Design review of the part built by this model. Coordinates are the model's own, in mm. Give positions to 0.01 mm unless a question says otherwise; leave off trailing zeros. Loops run counter-clockwise (first coordinate to the right, second up) from the corner with the lowest first, then second, coordinate; pieces in that order, holes last. Notation, with made-up numbers: (-32, -13.75) -> (-4, -13.75) arc R31 cw to (-4, 22.25) -> close; hole circle Ø9 at (88, -32). An arc over 180 degrees is marked (long way). Answer in a Markdown table with one row per item. Add a question column.
(1) For line 1 (Z direction, x = 1.2, y = -120.2); line 2 (Y direction, x = 1.7, z = -216.75); line 3 (Z direction, x = 1.35, y = 74), list the stretches that pass through material, from the lowest coordinate up.
(2) Consider section C-C on x = 1.5. Count the separate pieces of the cut face and the enclosed holes in it, then the cut area to 3 significant figures.
(3) For pin 1 (8 mm diameter, centred on y = -25, z = -216.75, fed in from -X); pin 2 (1 mm diameter, centred on x = 0.5, y = -47, fed in from +Z); pin 3 (1 mm diameter, centred on x = 1.5, y = 101, fed in from +Z); pin 4 (1 mm diameter, centred on x = 1.5, z = -155.5, fed in from +Y), all flat-tipped, find the tip position at first contact; note any pin that passes through.
(4) Draft analysis for pull direction Y (two halves, no side actions). For faces 1 (the flat face through (1.565, 23.665, -389.587)), 2 (the flat face through (1.57, -16.66, -150.86)), 3 (the flat face through (1.565, 0.768, -139.304)), 4 (the flat face through (0, -35, -255)), state which applies: +Y half, -Y half, draft (parallel to the pull), parting line (faces both ways), or undercut.
(5) Consider section D-D on y = 98. Write out the cut boundary in (x, z) (3 decimals).
(6) Consider section B-B on z = -279. Write out the cut boundary in (x, y) (3 decimals), then the cut area to 3 significant figures.
Autodesk Inventor part; units mm, degrees
ref_plane "YZ Plane" through (0, 0, 0) normal (1, 0, 0) x (0, 1, 0)
ref_plane "XZ Plane" through (0, 0, 0) normal (0, 1, 0) x (-1, 0, 0)
ref_plane "XY Plane" through (0, 0, 0) normal (0, 0, 1) x (1, 0, 0)
sketch "Sketch1" plane through (0, 0, 0) normal (1, 0, 0) x (0, 1, 0)
  line L0 (-120.8333, -99.25) -> (-47.8333, -99.25)
  line L1 (-120.2, -86.75) -> (-120.2, -99.25) construction
  line L2 (0, -198.5) -> (40, -198.5) construction
  line L3 (40, -198.5) -> (40, -265) construction
  line L4 (40, -265) -> (0, -265) construction
  line L5 (0, -265) -> (0, -198.5) construction
  line L6 (0, -265) -> (40, -265) construction
  line L7 (40, -265) -> (40, -285) construction
  line L8 (40, -285) -> (0, -285)
  line L9 (0, -285) -> (0, -265) construction
  line L10 (0, -198.5) -> (40, -198.5) construction
  line L11 (40, -198.5) -> (40, -178.5) construction
  line L12 (40, -178.5) -> (0, -178.5) construction
  line L13 (0, -178.5) -> (0, -198.5) construction
  line L14 (48.2, -259.95) -> (-8.2, -259.95) construction
  line L15 (-8.2, -259.95) -> (-8.2, -203.55) construction
  line L16 (-8.2, -203.55) -> (48.2, -203.55) construction
  line L17 (48.2, -203.55) -> (48.2, -259.95) construction
  line L18 (48.2, -231.75) -> (-8.2, -231.75) construction
  line L19 (40, -231.75) -> (0, -231.75) construction
  line L20 (43.57, -255.32) -> (-3.57, -255.32) construction
  line L21 (-3.57, -255.32) -> (-3.57, -208.18) construction
  line L22 (-3.57, -208.18) -> (43.57, -208.18) construction
  line L23 (43.57, -208.18) -> (43.57, -255.32) construction
  line L24 (43.57, -255.32) -> (48.2, -255.32) construction
  line L25 (43.57, -255.32) -> (43.57, -259.95) construction
  line L26 (-3.57, -208.18) -> (-8.2, -208.18) construction
  line L27 (-3.57, -208.18) -> (-3.57, -203.55) construction
  line L28 (40, -188.5) -> (0, -188.5) construction
  line L29 (40, -275) -> (0, -275) construction
  circle A0 centre (30, -275) radius 2.1
  circle A1 centre (10, -275) radius 2.1
  circle A2 centre (30, -188.5) radius 2.1
  circle A3 centre (10, -188.5) radius 2.1
  circle A4 centre (43.57, -255.32) radius 2.6
  circle A5 centre (43.57, -208.18) radius 2.6
  circle A6 centre (-3.57, -208.18) radius 2.6
  circle A7 centre (-3.57, -255.32) radius 2.6
  circle A8 centre (20, -231.75) radius 19.15
  circle A9 centre (-25, -216.75) radius 11.08 construction
  circle A10 centre (-25, -216.75) radius 13 construction
  circle A11 centre (-25, -216.75) radius 2.5
  line L30 (-60, -351.75) -> (-60, -111.75) construction
  circle A12 centre (-60, -111.75) radius 2.6
  circle A13 centre (-60, -351.75) radius 2.6
  line L31 (-120.2, -351.75) -> (-120.2, -111.75) construction
  circle A14 centre (-120.2, -111.75) radius 2.6
  circle A15 centre (-120.2, -351.75) radius 2.6
  circle A16 centre (-60, -111.75) radius 12 construction
  circle A17 centre (-120.2, -111.75) radius 12 construction
  circle A18 centre (-120.2, -351.75) radius 12 construction
  circle A19 centre (-60, -351.75) radius 12 construction
  circle A20 centre (-25, -246.75) radius 2.5
  circle A21 centre (-25, -246.75) radius 11.08 construction
  circle A22 centre (-25, -246.75) radius 13 construction
  circle A23 centre (20, -231.75) radius 11.08 construction
  circle A24 centre (20, -231.75) radius 13 construction
  line L32 (-23.1873, -227.6807) -> (18.1873, -220.8193) construction
  line L33 (18.1873, -242.6807) -> (-23.1873, -235.8193) construction
  line L34 (-47.8333, -364.25) -> (-120.8333, -364.25)
  line L35 (-132.8333, -352.25) -> (-132.8333, -111.25)
  line L36 (-60, -351.75) -> (-120.2, -351.75) construction
  line L37 (-120.2, -111.75) -> (-60, -111.75) construction
  line L38 (-60, -351.75) -> (-60, -364.25) construction
  line L39 (-120.2, -111.75) -> (-120.2, -99.25) construction
  line L40 (48.3276, -178.5) -> (48.3276, -285)
  line L41 (17.6122, -285) -> (40, -285) construction
  arc A25 (-132.8333, -352.25) -> (-120.8333, -364.25) centre (-120.8333, -352.25) ccw
  arc A26 (-120.8333, -99.25) -> (-132.8333, -111.25) centre (-120.8333, -111.25) ccw
  line L42 (48.3276, -178.5) -> (-47.8333, -99.25)
  line L43 (-47.8333, -364.25) -> (-47.8333, -99.25) construction
  line L44 (-120.2, -111.75) -> (-132.8333, -111.75) construction
  line L45 (-60, -351.75) -> (-47.8333, -351.75) construction
  line L46 (-36.08, -246.75) -> (-36.08, -485.113) construction
  line L47 (-47.8333, -344.25) -> (-47.8333, -285)
  line L48 (-47.8333, -285) -> (16.8804, -285)
  line L49 (-47.8333, -125.1668) -> (16.8804, -178.5)
  line L50 (-47.8333, -178.5) -> (16.8804, -178.5)
  line L51 (-47.8333, -125.1668) -> (-47.8333, -178.5)
  line L52 (48.3276, -285) -> (48.3276, -364.25)
  line L53 (48.3276, -364.25) -> (-47.8333, -364.25)
  line L54 (-47.8333, -344.25) -> (28.3276, -344.25)
  line L55 (28.3276, -344.25) -> (28.3276, -285)
  line L56 (-47.8333, -344.25) -> (28.3276, -285) construction
  line L57 (-39.6904, -344.25) -> (28.3276, -291.3349)
  line L58 (-47.8333, -337.9151) -> (20.1847, -285)
  line L59 (48.3276, -414.25) -> (124.3276, -414.25)
  line L60 (124.3276, -414.25) -> (124.3276, -364.25)
  line L61 (124.3276, -364.25) -> (48.3276, -364.25)
  line L62 (48.3276, -364.25) -> (48.3276, -414.25)
  line L63 (48.3276, -414.25) -> (-1.6724, -364.25)
  line L64 (98.3276, -364.25) -> (48.3276, -314.25)
  point P0 (-132.8333, -99.25)
  point P1 (28.3276, 86.5)
  point P2 (0, 86.5)
  point P3 (20.1847, 86.5)
  point P4 (20.1847, 86.5)
  point P5 (0, 86.5)
  point P6 (-132.8333, -364.25)
  point P7 (-47.8333, -338.3332)
  point P8 (0, -285)
  point P9 (48.3276, -364.25)
  dimension "d222" = 85
  dimension "d242" = 76
  dimension "d243" = 50
  dimension "d244" = 45
  dimension "d245" = 50
  dimension "d246" = 45
extrude "Extrusion1" add sketch "Sketch1" along normal blind 3.175 contours L0 L42 L40 L52 L53 L34 A25 L35 A26 | L62 L63 L53 | L61 L60 L59 L62 | L55 L57 L54 L47 L58 L8 | L58 L47 L48 L8 | L55 L54 L57 | A0 | A1 | A2 | A3 | A4 | A5 | A6 | A7 | A8
sketch "Sketch6" plane through (3.175, 0, 0) normal (1, 0, 0) x (0, 0, -1)
  line L0 (125.1668, -47.8333) -> (178.5, 16.8804)
  line L1 (291.3349, 28.3276) -> (344.25, 28.3276)
  line L2 (159.4204, -6.2705) -> (143.9864, 6.4492) construction
  line L3 (178.5, 48.3276) -> (99.25, -47.8333) construction
  line L4 (291.3349, 28.3276) -> (344.25, 28.3276) construction
  line L5 (317.7924, 28.3276) -> (317.7924, 48.3276) construction
  line L6 (364.25, 48.3276) -> (178.5, 48.3276) construction
  line L7 (151.7034, 0.0893) -> (161.2432, 11.6648) construction
  line L8 (151.7034, 0.0893) -> (142.1636, -11.4861) construction
  line L9 (317.7924, 38.3276) -> (302.7924, 38.3276) construction
  line L10 (317.7924, 38.3276) -> (332.7924, 38.3276) construction
  circle A0 centre (332.7924, 38.3276) radius 2.6
  circle A1 centre (302.7924, 38.3276) radius 2.6
  circle A2 centre (161.2432, 11.6648) radius 2.6
  circle A3 centre (142.1636, -11.4861) radius 2.6
  point P0 (414.25, 48.3276)
  point P1 (314.25, 48.3276)
  dimension "d233" = 15
  dimension "d234" = 15
  dimension "d235" = 15
  dimension "d236" = 15
  dimension "d237" = 5.2
  dimension "d238" = 5.2
  dimension "d239" = 5.2
  dimension "d240" = 5.2
  dimension "d241" = 30
extrude "Extrusion6" cut sketch "Sketch6" against normal through all
fillet "Fillet2" radius 3.175 5 edges at (1.5875, -47.8333, -125.1668) (1.5875, -47.8333, -178.5) (1.5875, 16.8804, -178.5) (1.5875, -47.8333, -99.25) (1.5875, 48.3276, -178.5)
fillet "Fillet3" radius 3.175 5 edges at (1.5875, 48.3276, -364.25) (1.5875, -1.6724, -364.25) (1.5875, 48.3276, -414.25) (1.5875, 124.3276, -414.25) (1.5875, 124.3276, -364.25)
sketch "Sketch7" plane through (3.175, 0, 0) normal (1, 0, 0) x (0, 0, -1)
  line L0 (414.25, 49.6427) -> (414.25, 121.1526) construction
  line L1 (414.25, 121.5776) -> (394.25, 121.5776) construction
  line L2 (394.25, 121.5776) -> (394.25, 71.5776) construction
  line L3 (394.25, 71.5776) -> (414.25, 71.5776) construction
  line L4 (414.25, 71.5776) -> (414.25, 121.5776) construction
  line L5 (404.25, 121.5776) -> (404.25, 71.5776) construction
  circle A0 centre (404.25, 106.5776) radius 2.6
  circle A1 centre (404.25, 86.5776) radius 2.6
  line L6 (411.075, 124.3276) -> (367.425, 124.3276)
  point P0 (0, 0)
  dimension "d248" = 20
  dimension "d249" = 50
  dimension "d250" = 5.2
  dimension "d251" = 5.2
  dimension "d252" = 15
  dimension "d253" = 15
  dimension "d256" = 2.75
extrude "Extrusion7" cut sketch "Sketch7" against normal up to next
sketch "Sketch8" plane through (3.175, 0, 0) normal (1, 0, 0) x (0, 0, -1)
  line L0 (302.7924, 28.3276) -> (332.7924, 28.3276) construction
  line L1 (332.7924, 28.3276) -> (332.7924, -26.6724) construction
  line L2 (332.7924, -26.6724) -> (302.7924, -26.6724) construction
  line L3 (302.7924, -26.6724) -> (302.7924, 28.3276) construction
  circle A0 centre (332.7924, 38.3276) radius 2.6
  circle A1 centre (302.7924, 38.3276) radius 2.6
  line L4 (332.7924, 38.3276) -> (302.7924, 38.3276) construction
  line L5 (317.7924, 38.3276) -> (317.7924, 28.3276) construction
  line L6 (328.7924, -26.6724) -> (306.7924, -26.6724) construction
  line L7 (306.7924, -26.6724) -> (306.7924, -6.6724) construction
  line L8 (306.7924, -6.6724) -> (328.7924, -6.6724) construction
  line L9 (328.7924, -6.6724) -> (328.7924, -26.6724) construction
  line L10 (312.7924, -11.6724) -> (322.7924, -11.6724) construction
  line L11 (322.7924, -11.6724) -> (322.7924, -21.6724) construction
  line L12 (322.7924, -21.6724) -> (312.7924, -21.6724) construction
  line L13 (312.7924, -21.6724) -> (312.7924, -11.6724) construction
  circle A2 centre (312.7924, -11.6724) radius 2.6
  circle A3 centre (322.7924, -21.6724) radius 2.6
  point P0 (0, 0)
  dimension "d257" = 30
  dimension "d258" = 55
  dimension "d259" = 10
  dimension "d260" = 22
  dimension "d261" = 20
  dimension "d262" = 4
  dimension "d263" = 10
  dimension "d264" = 10
  dimension "d265" = 5
  dimension "d266" = 6
  dimension "d267" = 5.2
  dimension "d268" = 5.2
extrude "Extrusion8" cut sketch "Sketch8" against normal up to next contours A2 | A3
sketch "Sketch9" plane through (3.175, 0, 0) normal (1, 0, 0) x (0, 0, -1)
  line L0 (45.8374, 19.9996) -> (577.1226, 19.9996) construction
  line L1 (361.075, 48.3276) -> (179.9977, 48.3276) construction
  line L2 (231.7502, 111.484) -> (231.7502, -169.9488) construction
  circle A0 centre (161.2432, 11.6648) radius 2.6
  circle A1 centre (231.7502, 19.9996) radius 3.5
  circle A2 centre (251.7502, 19.9996) radius 2.6
  circle A3 centre (211.7502, 19.9996) radius 2.6
  point P0 (0, 0)
  dimension "d271" = 28.328
  dimension "d272" = 70.507
  dimension "d273" = 7
  dimension "d274" = 5.2
  dimension "d275" = 20
  dimension "d276" = 5.2
  dimension "d277" = 20
extrude "Extrusion9" cut sketch "Sketch9" against normal up to next contours A1 | A2 | A3
properties part number "X Axis V Wheel RIGHT Outside Frame Machined"
Values follow:
| question | item | result |
|---|---|---|
| 1 | line 1 | -364.25 to -354.35, -349.15 to -114.35, -109.15 to -99.25 |
| 1 | line 2 | -132.83 to -27.5, -22.5 to 48.33 |
| 1 | line 3 | -414.25 to -364.25 |
| 2 | separate pieces | 1 |
| 2 | enclosed holes | 18 |
| 2 | area | 47,100 mm2 |
| 3 | pin 1 | x = 0 |
| 3 | pin 2 | z = -99.61 |
| 3 | pin 3 | z = -364.25 |
| 3 | pin 4 | y = 21.03 |
| 4 | face 1 | -Y half |
| 4 | face 2 | undercut |
| 4 | face 3 | +Y half |
| 4 | face 4 | draft |
| 5 | outline | (0, -414.25) -> (3.175, -414.25) -> (3.175, -364.25) -> (0, -364.25) -> close |
| 6 | outline | (0, -132.833) -> (3.175, -132.833) -> (3.175, 48.328) -> (0, 48.328) -> close |
| 6 | area | 575 mm2 |
